Work out the finished part from the listing and answer in its coordinate system (mm). Face numbers are marked on the shaded views. A direction names the side the tool comes from. Give positions to 0.01 mm unless a question says otherwise; leave off trailing zeros. Order: outer loops, then holes, each group sorted by start corner. A loop starts at its lowest first (then second) coordinate and runs counter-clockwise, first axis right, second up. Notation, with made-up numbers: (40.5, -25) - (77.5, -25) arc R31 ccw to (77.5, 3) - close; hole circle Ø3 at (82, 88.5). An arc over 180 degrees is marked (long way). Put each result on its own line as item: value.
```python
from build123d import *

# Parameters (mm, degrees)
PAD_DEPTH    = 22
POCKET_DEPTH = 20


with BuildPart() as part:
    # Sketch → Pad (new body)
    with BuildSketch(Plane.XY):
        Polygon((0.810902, 9.567203), (25.199765, 9.567203), (25.199765, 11.567203), (11.199765, 11.567203), (11.199765, 14.567203), (191.199765, 14.567203), (191.199765, 16.067203), (187.999779, 16.867203), (187.999779, 15.867203), (184.799779, 16.867203), (184.799779, 15.867203), (181.599779, 16.867203), (181.599779, 15.867203), (178.399779, 16.867203), (178.399779, 15.867203), (175.199779, 16.867203), (175.199779, 15.867203), (171.999779, 16.867203), (171.999779, 15.867203), (168.799779, 16.867203), (168.799779, 15.867203), (165.599779, 16.867203), (165.599779, 15.867203), (162.399779, 16.867203), (162.399779, 15.867203), (159.199779, 16.867203), (159.199779, 15.867203), (155.999779, 16.867203), (155.999779, 15.867203), (152.799779, 16.867203), (152.799779, 15.867203), (149.599779, 16.867203), (149.599779, 15.867203), (146.399779, 16.867203), (146.399779, 15.867203), (143.199779, 16.867203), (143.199779, 15.867203), (139.999779, 16.867203), (139.999779, 15.867203), (136.799779, 16.867203), (136.799779, 15.867203), (133.599779, 16.867203), (133.599779, 15.867203), (130.399779, 16.867203), (130.399779, 15.867203), (127.199779, 16.867203), (127.199779, 15.867203), (123.999779, 16.867203), (123.999779, 15.867203), (120.799779, 16.867203), (120.799779, 15.867203), (117.599779, 16.867203), (117.599779, 15.867203), (114.399779, 16.867203), (114.399779, 15.867203), (111.199779, 16.867203), (111.199779, 15.867203), (107.999779, 16.867203), (107.999779, 15.867203), (104.799779, 16.867203), (104.799779, 15.867203), (101.599779, 16.867203), (101.599779, 15.867203), (98.399779, 16.867203), (98.399779, 15.867203), (95.199779, 16.867203), (95.199779, 15.867203), (91.999779, 16.867203), (91.999779, 15.867203), (88.799779, 16.867203), (88.799779, 15.867203), (85.599779, 16.867203), (85.599779, 15.867203), (82.399779, 16.867203), (82.399779, 15.867203), (79.199779, 16.867203), (79.199779, 15.867203), (75.999779, 16.867203), (75.999779, 15.867203), (72.799779, 16.867203), (72.799779, 15.867203), (69.599779, 16.867203), (69.599779, 15.867203), (66.399779, 16.867203), (66.399779, 15.867203), (63.199779, 16.867203), (63.199779, 15.867203), (59.999772, 16.867203), (59.999772, 15.867203), (57.832203, 16.867203), (3.316658, 16.867203), (-12.582002, 0.001582), (-8.206291, 0.001582), align=None)
    extrude(amount=PAD_DEPTH)

    # Sketch001 (on Face91 of Pad) → Pocket (cut)
    with BuildSketch(Plane(origin=(0, 16.867203, 0), x_dir=(-1, 0, 0), z_dir=(0, 1, 0))):
        with BuildLine():
            ThreePointArc((-197.532818, 43.580935), (-210.073285, 31.040467), (-197.532818, 18.5))
            Line((-197.532818, 18.5), (-56.404323, 18.5))
            ThreePointArc((-56.404323, 18.5), (-43.863855, 31.040467), (-56.404323, 43.580935))
            Line((-197.532818, 43.580935), (-56.404323, 43.580935))
        make_face()
        with BuildLine():
            ThreePointArc((-197.532818, 3.5), (-210.073285, -9.040467), (-197.532818, -21.580935))
            Line((-197.532818, -21.580935), (-56.404323, -21.580935))
            ThreePointArc((-56.404323, -21.580935), (-43.863855, -9.040467), (-56.404323, 3.5))
            Line((-197.532818, 3.5), (-56.404323, 3.5))
        make_face()
    extrude(amount=-POCKET_DEPTH, mode=Mode.SUBTRACT)


solid = part.part
```
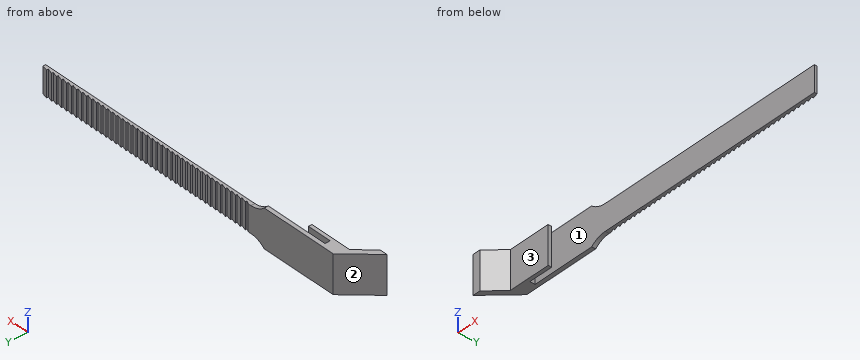
(1) Section A-A, the plane x = 13.5 is taken. Write down the section's boundary in (y, z), then the cut area to 3 significant figures.
Geometry check:
outline: (9.57, 0) - (11.57, 0) - (11.57, 22) - (9.57, 22) - close; (14.57, 0) - (16.87, 0) - (16.87, 22) - (14.57, 22) - close
area: 94.6 mm²
(2) Given pin 1 (1.1 mm diameter, centred on y = 16.5, z = 11, fed in from -X); pin 2 (0.8 mm diameter, centred on y = 16.5, z = 9.5, fed in from -X); pin 3 (6 mm diameter, centred on x = 26.5, z = 9, fed in from -Y), each flat-ended and moving along its own axis, determine where each tip first touches the part or whether it passes through.
Geometry check:
pin 1: stops at x = 2.45
pin 2: stops at x = 2.59
pin 3: stops at y = 9.57
(3) Straight lines are drawn through the part: line 1 (Y direction, x = 22.5, z = 3); line 2 (Y direction, x = 38, z = 8.75); line 3 (Z direction, x = 130, y = 15.25). For each, find the intervals that lie inside material, in ascending order.
Geometry check:
line 1: y = 9.57 to 11.57, 14.57 to 16.87
line 2: y = 14.57 to 16.87
line 3: z = 3.5 to 18.5
(4) Section B-B, the plane y = 4 is taken. Write down the section's boundary in (x, z), then the cut area to 3 significant figures.
Geometry check:
outline: (-8.81, 0) - (-4.44, 0) - (-4.44, 22) - (-8.81, 22) - close
area: 96.3 mm²
(5) A tool of negligible diameter and unlimited length cuts with its end or side. For the marked faces 1, 2 and 3, from which of +Z, -Z, +X, -X, +Y, -Y can it reach the whole face along a straight path? Write none if from no direction.
Geometry check:
face 1: +Z, -Z, +X
face 2: +Z, -Z, -X, +Y
face 3: +Z, -Z, +X, -Y
